Can you work these out from the model? Positions are in its coordinate system, mm. A direction names the side the tool comes from. Round coordinates to 2 decimals unless told otherwise and drop trailing zeros. Loops run counter-clockwise (first coordinate to the right, second up) from the corner with the lowest first, then second, coordinate; pieces in that order, holes last. Notation, with made-up numbers: (8, -22.5) -> (62, -22.5) arc R8 ccw to (62, -11.5) -> close; hole circle Ø6 at (87.25, -22). An arc over 180 degrees is marked (long way). Write item = value, one per line.
Autodesk Inventor part; units mm, degrees
ref_plane "YZ Plane" through (0, 0, 0) normal (1, 0, 0) x (0, 1, 0)
ref_plane "XZ Plane" through (0, 0, 0) normal (0, 1, 0) x (-1, 0, 0)
ref_plane "XY Plane" through (0, 0, 0) normal (0, 0, 1) x (1, 0, 0)
sketch "Sketch1" plane through (0, 0, 0) normal (0, 1, 0) x (-1, 0, 0)
  line L0 (0, 20) -> (-30, 20)
  line L1 (-30, 20) -> (-30, -20)
  line L2 (-30, -20) -> (0, -20)
  line L3 (0, -20) -> (0, 20)
  point P0 (0, 0)
  dimension "d0" = 20
  dimension "d1" = 20
  dimension "d2" = 0
  dimension "d3" = 30
extrude "Plate1" add sketch "Sketch1" along normal blind 2
sketch "Sketch3" plane through (29.316, 1.8794, -20) normal (0.3420201, -0.9396926, 0) x (0.9396926, 0.3420201, 0)
  line L0 (0, 40) -> (0, 0)
  line L1 (0, 0) -> (25, 0)
  line L2 (25, 0) -> (25, 40)
  line L3 (25, 40) -> (0, 40)
edge flange "Flange1" height 25 angle 20 thickness 2 bend radius 2 thickness toward (0.3420201, -0.9396926, 0) relief tear relief width 2 relief depth 1 edges at (30, 2, 0) wall of the first edge with corners at (29.316, 1.8794, 20) (29.316, 1.8794, -20) (52.8083, 10.4299, -20) (52.8083, 10.4299, 20)
bend "Bend1"
corner "Corner1"
sketch "Sketch4" plane through (52.8083, 10.4299, 20) normal (-0.3420201, 0.9396926, 0) x (0.9396926, 0.3420201, 0)
  line L0 (-24.2947, 40) -> (-24.2947, 0)
  line L1 (-24.2947, 0) -> (0, 0)
  line L2 (0, 0) -> (0, 40)
  line L3 (-24.2947, 40) -> (0, 40)
  line L4 (-24.2947, -67.5) -> (0, -67.5)
  line L5 (0, -67.5) -> (0, 107.5)
  line L6 (0, 107.5) -> (-24.2947, 107.5)
  line L7 (-24.2947, 107.5) -> (-24.2947, -67.5)
  point P0 (-53.1908, 20)
  dimension "d19" = 67.5
  dimension "d20" = 67.5
  dimension "d21" = 0
  dimension "d22" = 0
extrude "Extrusion1" add sketch "Sketch4" against normal blind 2 contours L7 L6 L5 L3 | L1 L5 L4 L7
fillet "Fillet1" radius 2 2 edges at (0, 1, 20) (0, 1, -20)
fillet "Fillet2" radius 2 4 edges at (30.3208, 1.1809, 87.5) (53.1503, 9.4902, 87.5) (53.1503, 9.4902, -87.5) (30.3208, 1.1809, -87.5)
sketch "Sketch5" plane through (0, 2, 0) normal (0, 1, 0) x (1, 0, 0)
  circle A0 centre (15, 0) radius 3
  point P0 (0, 0)
  dimension "d44" = 6
  dimension "d45" = 15
  dimension "d46" = 0
extrude "Extrusion2" cut sketch "Sketch5" against normal blind 2
sketch "Sketch6" plane through (29.9787, 2.1206, 20) normal (-0.3420201, 0.9396926, 0) x (0.9396926, 0.3420201, 0)
  circle A0 centre (12, -59.5) radius 3.5
  arc A1 (2, 107.5) -> (0, 105.5) centre (2, 105.5) ccw
  line L0 (0, 105.5) -> (0, 40)
  line L1 (0, 40) -> (0, 0)
  line L2 (0, 0) -> (0, -65.5)
  arc A2 (0, -65.5) -> (2, -67.5) centre (2, -65.5) ccw
  line L3 (2, -67.5) -> (22.2947, -67.5)
  arc A3 (22.2947, -67.5) -> (24.2947, -65.5) centre (22.2947, -65.5) ccw
  line L4 (24.2947, -65.5) -> (24.2947, 105.5)
  arc A4 (24.2947, 105.5) -> (22.2947, 107.5) centre (22.2947, 105.5) ccw
  line L5 (22.2947, 107.5) -> (2, 107.5)
  circle A5 centre (12, 100.5) radius 3.5
  point P0 (-28.8961, 20)
  dimension "d32" = 7
  dimension "d35" = 160
  dimension "d40" = 8
  dimension "d41" = 12
extrude "Extrusion3" cut sketch "Sketch6" against normal blind 2 contours A0 | A5
equation "\"d20\" = d19"
equation "\"BendRadius\" = Thickness"
equation "\"BendReliefWidth\" = Thickness"
equation "\"BendReliefDepth\" = 0.5 * Thickness"
equation "\"CornerReliefSize\" = 4 * Thickness"
equation "\"MinimumRemnant\" = 2 * Thickness"
equation "\"TransitionRadius\" = BendRadius"
equation "\"JacobiRadiusSize\" = BendRadius"
equation "\"GapSize\" = Thickness"
properties part number "Top Mount" material "Stainless Steel"
1. Suppose I cut it at D-D, the plane z = 62. List the corners of the cut face in (x, y) for me.
Entries:
outline = (29.98, 2.12) -> (30.66, 0.24) -> (53.49, 8.55) -> (52.81, 10.43) -> close
2. I'm going to push flat-ended pins straight in: pin 1 (1.7 mm diameter, centred on x = 15.5, y = 0.5, fed in from -Z); pin 2 (0.6 mm diameter, centred on x = 23, y = 0.5, fed in from +Z); pin 3 (10 mm diameter, centred on x = 6, z = 23, fed in from +Y). Where does each tip first touch, or does it pass through?
Entries:
pin_1 = -20
pin_2 = 20
pin_3 = 2
3. I need wall thicknesses on line 1 (Z direction, x = 15, y = 0.5); line 2 (Y direction, x = 19.5, z = 7); line 3 (Z direction, x = 8, y = 1.75). Which ranges of each line are inside material? Lowest first, please. Write a range as [from, to].
Entries:
line_1 = [-20, -3], [3, 20]
line_2 = [0, 2]
line_3 = [-20, 20]
4. For faces 5 (the flat face through (42, 5, -87.5)), 6 (the flat face through (11.6, 2, 0.3)), which set-ups out of +Z, -Z, +X, -X, +Y, -Y let a thin tool reach every point of the face, with its end or its side?
Entries:
face_5 = -Z, +X, -X, +Y, -Y
face_6 = +Z, -Z, -X, +Y
5. Suppose I cut it at C-C, the plane x = 6. List the corners of the cut face in (y, z) for me, and give its area (3 significant figures).
Entries:
outline = (0, -20) -> (2, -20) -> (2, 20) -> (0, 20) -> close
area = 80.0 mm²
6. Suppose I cut it at A-A, the plane x = 15. List the corners of the cut face in (y, z) for me.
Entries:
outline = (0, -20) -> (2, -20) -> (2, -3) -> (0, -3) -> close; (0, 3) -> (2, 3) -> (2, 20) -> (0, 20) -> close
7. We'd pull the mould along Z, two halves only. Please class faces 1 (the flat face through (11.6, 0, 0.3)), 2 (the cylindrical face through (40.879, 5.039, 82.917)), 3 (the cylindrical face through (12, 1, 0)), 4 (the flat face through (42, 5, 87.5)): released by +Z, released by -Z, zero draft, split by the parting line, or undercut.
Entries:
face_1 = zero draft
face_2 = undercut
face_3 = undercut
face_4 = released by +Z
8. Suppose I cut it at B-B, the plane z = 0. List the corners of the cut face in (x, y) for me, and give its area (3 significant figures).
Entries:
outline = (0, 0) -> (12, 0) -> (12, 2) -> (0, 2) -> close; (18, 0) -> (29.29, 0) arc R4 ccw to (30.66, 0.24) -> (53.49, 8.55) -> (52.81, 10.43) -> (29.98, 2.12) arc R2 cw to (29.29, 2) -> (18, 2) -> close
area = 97.3 mm²
